Input: part model. Units: mm. Frame: model coordinates. Face numbers are marked on the shaded views. A direction names the side the tool comes from. Coordinates: 2 decimals unless noted, no trailing zeros. Loops run counter-clockwise (first coordinate to the right, second up) from the corner with the lowest first, then second, coordinate; pieces in that order, holes last. Notation, with made-up numbers: (47, 49) - (77, 49) arc R32 ccw to (77, 77) - close; hole circle Ø5 at (15.5, 68). An arc over 180 degrees is marked (long way). Use one line per item in the form item = value.
from build123d import *

# Parameters (mm, degrees)
SKETCH1_W                = 65
SKETCH1_H                = 130
MAIN_BODY_EXTRUDE_DEPTH  = 11
SKETCH4_R                = 5
BOLT_HOLES_DEPTH         = 11
UNDERCARRIAGE_CUT_DEPTH  = 135
TOP_CORNER_CUTS_DEPTH    = 11
BOTTOM_CORNER_CUTS_DEPTH = 11
TOP_CUT_DEPTH            = 130


with BuildPart() as part:
    # Sketch1 → Main Body Extrude (new body)
    with BuildSketch(Plane.XY):
        Rectangle(SKETCH1_W, SKETCH1_H)
    extrude(amount=MAIN_BODY_EXTRUDE_DEPTH)

    # Sketch4 → Bolt Holes (cut)
    with BuildSketch(Plane.XY.offset(11)):
        with Locations((0, -51)):
            Circle(SKETCH4_R)
        with Locations((0, -32.5)):
            Circle(SKETCH4_R)
        with Locations((0, 43)):
            Circle(SKETCH4_R)
        with BuildLine():
            Line((-5, -14), (-5, 24.5))
            ThreePointArc((-5, 24.5), (0, 29.5), (5, 24.5))
            Line((5, 24.5), (5, -14))
            ThreePointArc((5, -14), (0, -19), (-5, -14))
        make_face()
    extrude(amount=-BOLT_HOLES_DEPTH, mode=Mode.SUBTRACT)

    # Sketch6 → Undercarriage Cut (cut)
    with BuildSketch(Plane(origin=(0, 65, 0), x_dir=(1, 0, 0), z_dir=(0, 1, 0))):
        Polygon((21, -11), (18, -7), (18, -6), (32.5, -6), (32.5, -11), align=None)
        Polygon((-32.5, -11), (-21, -11), (-18, -7), (-18, -6), (-32.5, -6), align=None)
    extrude(amount=-UNDERCARRIAGE_CUT_DEPTH, mode=Mode.SUBTRACT)

    # Sketch2 → Top Corner Cuts (cut)
    with BuildSketch(Plane.XY.offset(11)):
        Polygon((-32.5, 55), (-17.5, 65), (-32.5, 65), align=None)
        Polygon((17.5, 65), (32.5, 55), (32.5, 65), align=None)
    extrude(amount=-TOP_CORNER_CUTS_DEPTH, mode=Mode.SUBTRACT)

    # Sketch3 → Bottom Corner Cuts (cut)
    with BuildSketch(Plane.XY.offset(11)):
        Polygon((-26.5, -65), (-32.5, -59), (-32.5, -65), align=None)
        Polygon((26.5, -65), (32.5, -59), (32.5, -65), align=None)
    extrude(amount=-BOTTOM_CORNER_CUTS_DEPTH, mode=Mode.SUBTRACT)

    # Sketch7 → Top Cut (cut)
    with BuildSketch(Plane(origin=(0, -65, 0), x_dir=(-1, 0, 0), z_dir=(0, -1, 0))):
        Polygon((24.5, 0), (-24.5, 0), (-24, -1), (24, -1), align=None)
    extrude(amount=-TOP_CUT_DEPTH, mode=Mode.SUBTRACT)


solid = part.part
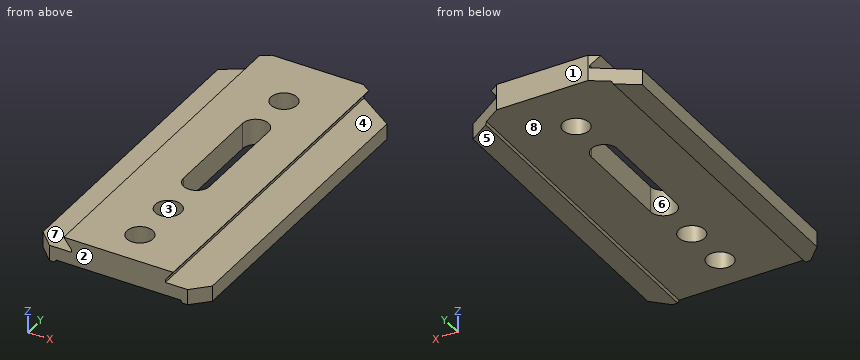
Q1. First-contact query: P1, Ø16, axis at x = 0, y = -32.5, coming from the -Z side; P2, Ø1.5, axis at y = 13, z = 7.5, coming from the -X side; P3, Ø0.8, axis at y = 12, z = 6.5, coming from the -X side. Flat tips, straight axial feed; report the tip coordinate or a pass-through.
Check values:
P1 = 1
P2 = -18.94
P3 = -18
Q2. Cut plane C-C, the plane x = 12. Return loops of the section in (y, z).
Check values:
outline = (-65, 1) - (65, 1) - (65, 11) - (-65, 11) - close
Q3. Cut plane A-A, the plane y = 43. Return loops of the section in (x, z), then the cut area to 4 significant figures.
Check values:
outline = (-32.5, 0) - (-24.5, 0) - (-24, 1) - (-5, 1) - (-5, 11) - (-21, 11) - (-18, 7) - (-18, 6) - (-32.5, 6) - close; (5, 1) - (24, 1) - (24.5, 0) - (32.5, 0) - (32.5, 6) - (18, 6) - (18, 7) - (21, 11) - (5, 11) - close
area = 433.5 mm²
Q4. Cut plane B-B, the plane x = 0. Return loops of the section in (y, z), then the cut area to 3 significant figures.
Check values:
outline = (-65, 1) - (-56, 1) - (-56, 11) - (-65, 11) - close; (-46, 1) - (-37.5, 1) - (-37.5, 11) - (-46, 11) - close; (-27.5, 1) - (-19, 1) - (-19, 11) - (-27.5, 11) - close; (29.5, 1) - (38, 1) - (38, 11) - (29.5, 11) - close; (48, 1) - (65, 1) - (65, 11) - (48, 11) - close
area = 515 mm²
Q5. Ray query, line 1 along Y through (x, z) = (0, 4.75); line 2 along X through (y, z) = (3, 1.5); line 3 along X through (y, z) = (20, 6.25). Return the intervals inside material, ascending. Write a range as [from, to].
Check values:
line_1 = [-65, -56], [-46, -37.5], [-27.5, -19], [29.5, 38], [48, 65]
line_2 = [-32.5, -5], [5, 32.5]
line_3 = [-18, -5], [5, 18]
Q6. Set-up query: the marked faces 4, 5, 6, 7 and 8. Return all of +Z, -Z, +X, -X, +Y, -Y with unobstructed straight access to the full face (end or side cutting, diameter ignored); none if empty.
Check values:
face_4 = +X, +Y, -Y
face_5 = -Z, +X, -X, +Y, -Y
face_6 = +Z, -Z
face_7 = -X, +Y, -Y
face_8 = -Z, +Y, -Y
Q7. Pull-direction query (Y, two-part tool) for the marked faces 1, 2 and 3; classes: pulls with the +Y half, pulls with the -Y half, needs draft (parallel to the pull), parting line crosses it, or undercut.
Check values:
face_1 = pulls with the +Y half
face_2 = pulls with the -Y half
face_3 = undercut
